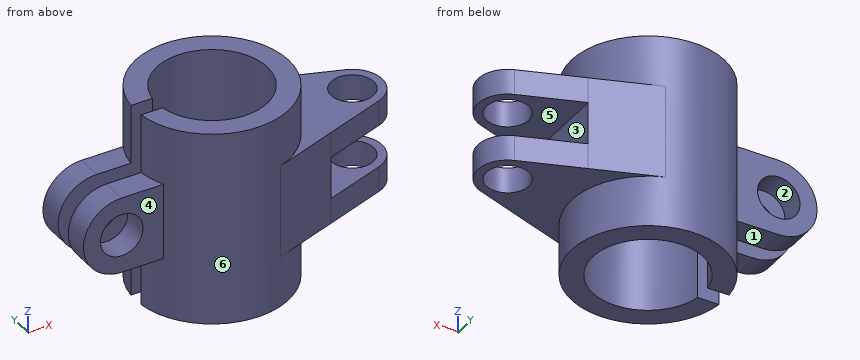
```python
from build123d import *

# Parameters (mm, degrees)
BOSS_EXTRUDE1_DEPTH = 46
BOSS_EXTRUDE2_START = 12
SKETCH1_3_R         = 5
BOSS_EXTRUDE2_DEPTH = 6
BOSS_EXTRUDE3_START = 28
SKETCH1_4_R         = 5
BOSS_EXTRUDE3_DEPTH = 6
BOSS_EXTRUDE4_START = 14
BOSS_EXTRUDE4_DEPTH = 18
FILLET2_RADIUS      = 9
FILLET2_LENGTH      = 6
FILLET3_RADIUS      = 9
FILLET3_LENGTH      = 6
BOSS_EXTRUDE5_START = 12
BOSS_EXTRUDE5_DEPTH = 22


with BuildPart() as part:
    # Sketch1 → Boss-Extrude1 (new body)
    with BuildSketch(Plane.XY):
        with BuildLine():
            ThreePointArc((-12.845232579, -2), (13, 0), (-12.845232579, 2))
            Line((-12.845232579, 2), (-17.88854382, 2))
            ThreePointArc((-17.88854382, 2), (18, 0), (-17.88854382, -2))
            Line((-17.88854382, -2), (-12.845232579, -2))
        make_face()
    extrude(amount=BOSS_EXTRUDE1_DEPTH)

    # Sketch1<5> → Boss-Extrude4 (add)
    with BuildSketch(Plane.XY.offset(BOSS_EXTRUDE4_START)):
        with BuildLine():
            Line((-35, 2), (-17.88854382, 2))
            ThreePointArc((-17.88854382, 2), (-17.269106839, 5.077198931), (-16.124515497, 8))
            Line((-16.124515497, 8), (-35, 8))
            Line((-35, 8), (-35, 2))
        make_face()
        with BuildLine():
            ThreePointArc((-16.124515497, -8), (-17.269106839, -5.077198931), (-17.88854382, -2))
            Line((-17.88854382, -2), (-35, -2))
            Line((-35, -2), (-35, -8))
            Line((-35, -8), (-16.124515497, -8))
        make_face()
    extrude(amount=BOSS_EXTRUDE4_DEPTH)

    # Fillet2: full round fillet: the end face becomes a half cylinder, R = half its width
    fillet2_face = Plane((-35, 5, 23), x_dir=(0, 1, 0), z_dir=(-1, 0, 0))  # on the end face: x along it, z out of the body
    fillet2_slab = fillet2_face.offset(-FILLET2_RADIUS / 2) * Box(FILLET2_LENGTH, 2 * FILLET2_RADIUS, FILLET2_RADIUS, mode=Mode.PRIVATE)  # the body's end, R deep
    fillet2_round = Plane((-26, 5, 23), x_dir=(-1, 0, 0), z_dir=(0, 1, 0)) * Cylinder(FILLET2_RADIUS, FILLET2_LENGTH, mode=Mode.PRIVATE)  # its axis R under the face
    add(fillet2_slab - fillet2_round, mode=Mode.SUBTRACT)

    # Fillet3: full round fillet: the end face becomes a half cylinder, R = half its width
    fillet3_face = Plane((-35, -5, 23), x_dir=(0, -1, 0), z_dir=(-1, 0, 0))  # on the end face: x along it, z out of the body
    fillet3_slab = fillet3_face.offset(-FILLET3_RADIUS / 2) * Box(FILLET3_LENGTH, 2 * FILLET3_RADIUS, FILLET3_RADIUS, mode=Mode.PRIVATE)  # the body's end, R deep
    fillet3_round = Plane((-26, -5, 23), x_dir=(-1, 0, 0), z_dir=(0, -1, 0)) * Cylinder(FILLET3_RADIUS, FILLET3_LENGTH, mode=Mode.PRIVATE)  # its axis R under the face
    add(fillet3_slab - fillet3_round, mode=Mode.SUBTRACT)

    # Sketch2 → Ø10.0mm Dowel Hole1 (revolve, cut)
    with BuildSketch(Plane(origin=(-26, 8, 23), x_dir=(0, 0, 1), z_dir=(1, 0, 0))):
        Polygon((0, 0), (0, 33.004303095), (5, 30), (5, 0), align=None)
    revolve(axis=Axis((-26, 14.35, 23), (0, -1, 0)), mode=Mode.SUBTRACT)



with BuildPart() as body_2:
    # Sketch1<3> → Boss-Extrude2 (new body)
    with BuildSketch(Plane.XY.offset(BOSS_EXTRUDE2_START)):
        with BuildLine():
            Line((35.333333333, 6.599663291), (21, 11.66726189))
            Line((21, 11.66726189), (21, -11.66726189))
            Line((21, -11.66726189), (35.333333333, -6.599663291))
            ThreePointArc((35.333333333, -6.599663291), (40, 0), (35.333333333, 6.599663291))
        make_face()
        with Locations((33, 0)):
            Circle(SKETCH1_3_R, mode=Mode.SUBTRACT)
    extrude(amount=BOSS_EXTRUDE2_DEPTH)


with BuildPart() as body_3:
    # Sketch1<4> → Boss-Extrude3 (new body)
    with BuildSketch(Plane.XY.offset(BOSS_EXTRUDE3_START)):
        with BuildLine():
            Line((35.333333333, 6.599663291), (21, 11.66726189))
            Line((21, 11.66726189), (21, -11.66726189))
            Line((21, -11.66726189), (35.333333333, -6.599663291))
            ThreePointArc((35.333333333, -6.599663291), (40, 0), (35.333333333, 6.599663291))
        make_face()
        with Locations((33, 0)):
            Circle(SKETCH1_4_R, mode=Mode.SUBTRACT)
    extrude(amount=BOSS_EXTRUDE3_DEPTH)


with BuildPart() as part_1:
    add(part.part)

    add(body_2.part)  # Boss-Extrude5 merges body 2

    add(body_3.part)  # Boss-Extrude5 merges body 3
    # Sketch1<6> → Boss-Extrude5 (add)
    with BuildSketch(Plane.XY.offset(BOSS_EXTRUDE5_START)):
        with BuildLine():
            Line((21, 11.66726189), (6, 16.970562748))
            ThreePointArc((6, 16.970562748), (18, 0), (6, -16.970562748))
            Line((6, -16.970562748), (21, -11.66726189))
            Line((21, -11.66726189), (21, 11.66726189))
        make_face()
    extrude(amount=BOSS_EXTRUDE5_DEPTH)


solid = part_1.part
```
For this review, take the finished solid that the model builds, in its own axes (mm). Face numbers are marked on the shaded views. A direction names the side the tool comes from. Give positions to 0.01 mm unless a question says otherwise; leave off trailing zeros. Write each loop counter-clockwise with the first axis right and the second up, starting at its lowest first coordinate (ties: lowest second). Pieces come first, ordered by that corner, then holes. Notation, with made-up numbers: M -24.5,86.5 L 18.5,86.5 A30 cw 18.5,114.5 Z; hole C 36.5,51 d4. An arc over 180 degrees is marked long. Answer as a JSON object with one key per item and string values. Group by question number.
Item 1: Tool access review of the marked faces 4, 5 and 6: name each direction out of +Z, -Z, +X, -X, +Y, -Y from which nothing blocks a thin tool from reaching the whole face with its end or side.
Item 2: Consider section C-C on z = 23. Write out the cut boundary in (x, y).
Item 3: For pin 1 Ø9 at (x, z) = (-30, 19.5) entering from +Y; pin 2 Ø1.8 at (x, y) = (-21.5, 5.5) entering from +Z; pin 3 Ø11.5 at (x, y) = (33, 0) entering from +Z; pin 4 Ø9 at (x, y) = (33, 0) entering from -Z, all flat-tipped, find the tip position at first contact; note any pin that passes through.
Item 4: For probe 1 along Y at (x, z) = (-0.5, 16); probe 2 along Z at (x, y) = (-26, 3.8); probe 3 along X at (y, z) = (0.5, 25), list the stretches that pass through material, from the lowest coordinate up. Write a range as [from, to].
Item 5: Consider section A-A on y = 0. Write out the cut boundary in (x, z).
Item 6: Consider section B-B on x = 0. Write out the cut boundary in (y, z).
Item 7: Consider section D-D on z = 33. Write out the cut boundary in (x, y).
Item 8: Draft analysis for pull direction X (two halves, no side actions). For the marked faces 1, 2 and 3, state which applies: +X half, -X half, draft (parallel to the pull), parting line (faces both ways), or undercut.
Check result:
{
 "1": {"face 4": "+Z, -Z, -X, -Y", "face 5": "+X, +Y, -Y", "face 6": "none"},
 "2": {"outline": "M -35,-8 L -31,-8 L -31,-2 L -35,-2 Z; M -35,2 L -31,2 L -31,8 L -35,8 Z; M -21,-8 L -16.12,-8 A18 ccw 6,-16.97 L 21,-11.67 L 21,11.67 L 6,16.97 A18 ccw -16.12,8 L -21,8 L -21,2 L -12.85,2 A13 cw long -12.85,-2 L -21,-2 Z"},
 "3": {"pin 1": "stops at y = 8", "pin 2": "stops at z = 32", "pin 3": "stops at z = 34", "pin 4": "passes through"},
 "4": {"probe 1": "y = [-17.99, -12.99], [12.99, 17.99]", "probe 2": "z = [14, 18], [28, 32]", "probe 3": "x = [12.99, 21]"},
 "5": {"outline": "M 13,0 L 18,0 L 18,12 L 28,12 L 28,18 L 21,18 L 21,28 L 28,28 L 28,34 L 18,34 L 18,46 L 13,46 Z; M 38,12 L 40,12 L 40,18 L 38,18 Z; M 38,28 L 40,28 L 40,34 L 38,34 Z"},
 "6": {"outline": "M -18,0 L -13,0 L -13,46 L -18,46 Z; M 13,0 L 18,0 L 18,46 L 13,46 Z"},
 "7": {"outline": "M -17.89,-2 A18 ccw 6,-16.97 L 35.33,-6.6 A7 ccw 35.33,6.6 L 6,16.97 A18 ccw -17.89,2 L -12.85,2 A13 cw long -12.85,-2 Z; hole C 33,0 d10"},
 "8": {"face 1": "draft", "face 2": "undercut", "face 3": "+X half"}
}
